Part print with two shaded views. Sizes in mm from the minimum x, y, z corner. A direction names the side the tool comes from. Give positions to 0.01 mm unless a question says otherwise; leave off trailing zeros. Write each loop counter-clockwise with the first axis right and the second up, starting at its lowest first coordinate (ties: lowest second). Pieces come first, ordered by that corner, then holes. Notation, with made-up numbers: (81.5, 3.5) -> (98.5, 3.5) arc R19 ccw to (98.5, 39.5) -> close; hole circle Ø5 at (50, 9.25). An arc over 180 degrees is marked (long way). Write item = value, one per line. Start each with the question number.
Q1. Drop flat-ended pins along their axis: P1, Ø8, axis at x = 158.5, z = 53, coming from the +Y side (1 decimal); P2, Ø1, axis at x = 77, y = 58, coming from the +Z side (1 decimal); P3, Ø10, axis at x = 159.5, y = 51, coming from the -Z side. Give the stop position or say it passes through.
Q2. Wall check: line 1 (X direction, y = 61, z = 31.5); line 2 (Z direction, x = 120, y = 34); line 3 (X direction, y = 35, z = 55). Give the ranges that are in metal, low to high.
Q3. Tool access for the marked faces 1 and 2: list every direction of +Z, -Z, +X, -X, +Y, -Y with a clear straight run to the whole face (end or side of a thin tool).
Q4. Saw through at C-C, the plane z = 13. List the corners of the cut face in (x, y), then the cut area to 3 significant figures.
Q5. Saw through at A-A, the plane y = 32.5. List the corners of the cut face in (x, z).
Q6. Saw through at B-B, the plane z = 32.5. List the corners of the cut face in (x, y).
Q7. Mould opens along Z. For the marked faces 3, 4 and 5 say: pulls with the +Z half, pulls with the -Z half, needs draft (parallel to the pull), parting line crosses it, or undercut.
Q8. Saw through at D-D, the plane x = 220. List the corners of the cut face in (y, z), then the cut area to 3 significant figures.
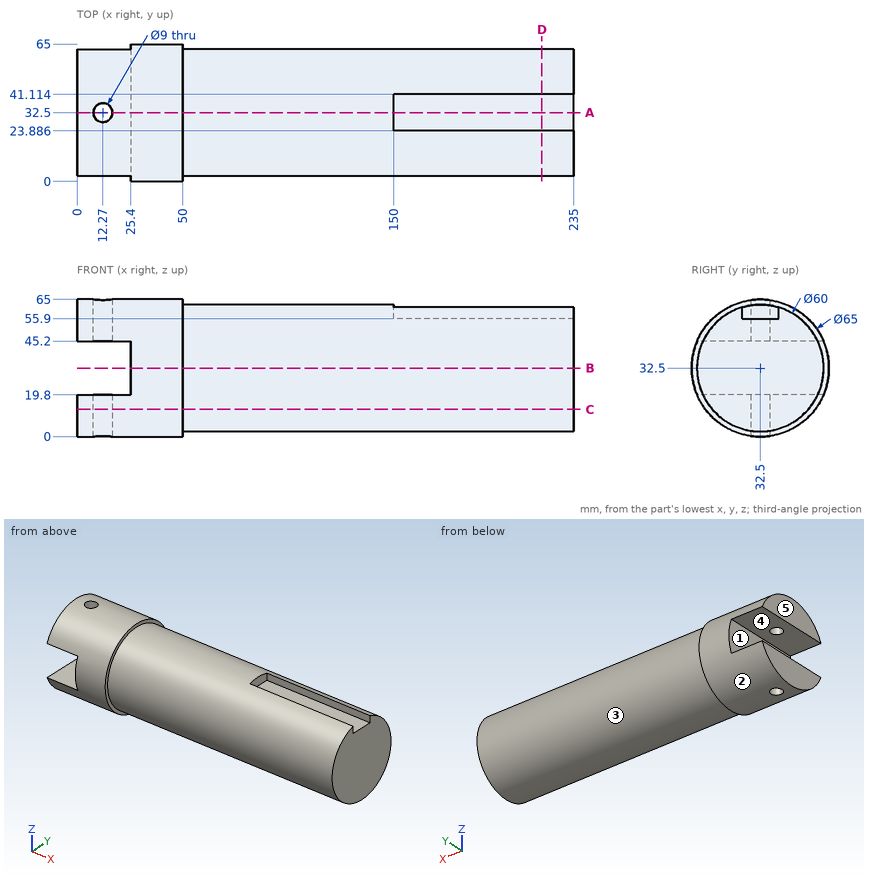
Report:
q1.P1 = 57.6
q1.P2 = 49.1
q1.P3 = 5.71
q2.line_1 = 25.4 to 235
q2.line_2 = 2.54 to 62.46
q2.line_3 = 0 to 8.53, 16.01 to 235
q3.face_1 = -X, +Y, -Y
q3.face_2 = +X, -X
q4.outline = (0, 6.5) -> (50, 6.5) -> (50, 9.7) -> (235, 9.7) -> (235, 55.3) -> (50, 55.3) -> (50, 58.5) -> (0, 58.5) -> close; hole circle Ø9 at (12.27, 32.5)
q4.area = 11,000 mm2
q5.outline = (0, 0) -> (7.77, 0) -> (7.77, 19.8) -> (0, 19.8) -> close; (0, 45.2) -> (7.77, 45.2) -> (7.77, 65) -> (0, 65) -> close; (16.77, 0) -> (50, 0) -> (50, 2.5) -> (235, 2.5) -> (235, 55.9) -> (150, 55.9) -> (150, 62.5) -> (50, 62.5) -> (50, 65) -> (16.77, 65) -> (16.77, 45.2) -> (25.4, 45.2) -> (25.4, 19.8) -> (16.77, 19.8) -> close
q6.outline = (25.4, 0) -> (50, 0) -> (50, 2.5) -> (235, 2.5) -> (235, 62.5) -> (50, 62.5) -> (50, 65) -> (25.4, 65) -> close
q7.face_3 = parting line crosses it
q7.face_4 = undercut
q7.face_5 = needs draft
q8.outline = (23.89, 55.9) -> (23.89, 61.24) arc R30 ccw (long way) to (41.11, 61.24) -> (41.11, 55.9) -> close
q8.area = 2,720 mm2
